Verification items for this drawing (mm, ordinates from the low corner). A direction names the side the tool comes from. Give positions to 0.01 mm unless a question says otherwise; leave off trailing zeros. Loops run counter-clockwise (first coordinate to the right, second up) from the corner with the lowest first, then second, coordinate; pieces in that order, holes last. Notation, with made-up numbers: (51.25, -15) -> (82.25, -15) arc R20 cw to (82.25, 6) -> close; hole circle Ø7 at (-32.5, 9.25). An arc over 180 degrees is marked (long way). Write item = value, one per line.
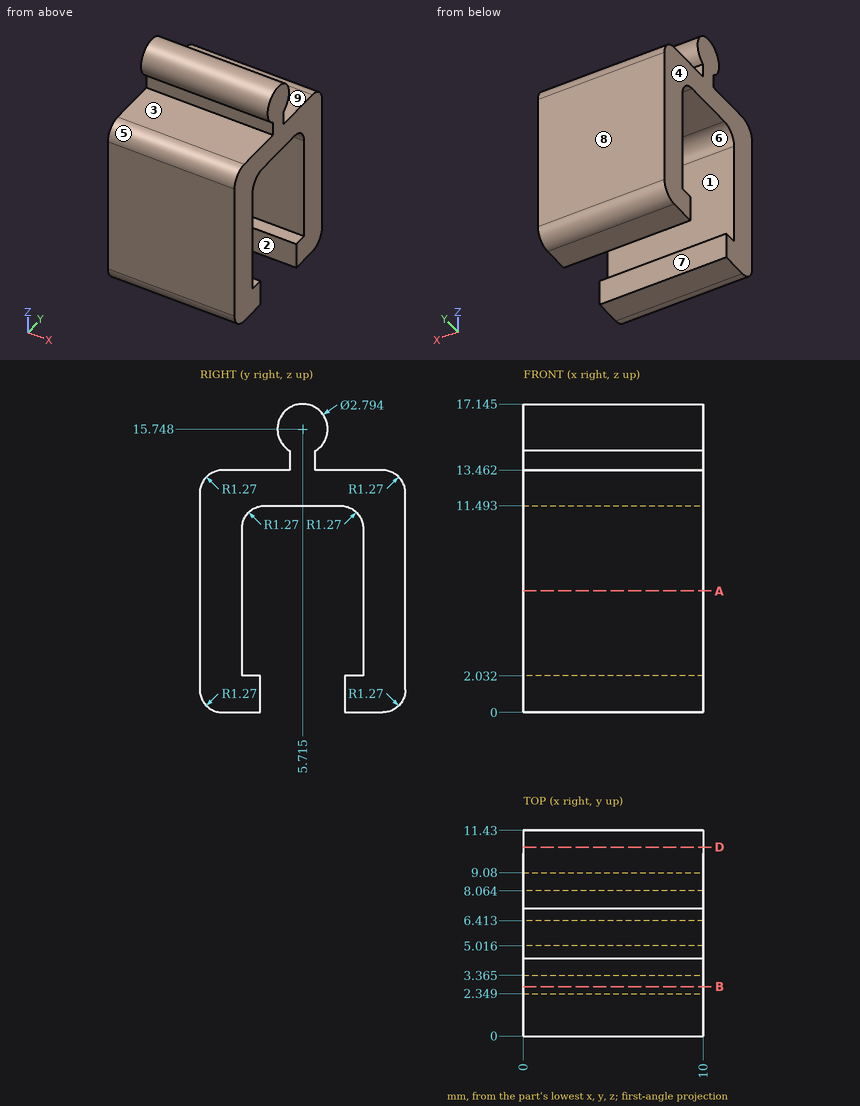
Item 1: Draft check along Y on the marked faces 6, 7, 8 and 9. Enter one of: +Y half, -Y half, draft (parallel to the pull), parting line (faces both ways), or undercut.
Answer:
face_6 = undercut
face_7 = undercut
face_8 = +Y half
face_9 = draft
Item 2: Gauge pin test, flat ends, axial feed: pin 1 (2 mm diameter, centred on x = 9, y = 7.5, fed in from +Z) (1 decimal); pin 2 (1.3 mm diameter, centred on x = 6, y = 6, fed in from -Z); pin 3 (1.1 mm diameter, centred on x = 7.5, y = 2.5, fed in from +Z); pin 4 (6 mm diameter, centred on y = 4.5, z = 11.5, fed in from -X). Record the tip position at first contact, or that the pin passes through.
Answer:
pin_1 = 16.9
pin_2 = 11.49
pin_3 = 13.46
pin_4 = 0
Item 3: Thickness scan on L1, parallel to Y at x = 5, z = 5.75; L2, parallel to Y at x = 5.25, z = 1.5 (1 decimal); L3, parallel to Z at x = 4.75, y = 9.5. Record the ranges inside material, lowest first. Write a range as [from, to].
Answer:
L1 = [0, 2.35], [9.08, 11.43]
L2 = [0, 3.4], [8.1, 11.4]
L3 = [0, 13.46]
Item 4: Section check D-D, the plane y = 10.5. Record the cut outline in (x, z) (1 decimal), plus the area to 3 significant figures.
Answer:
outline = (0, 0) -> (10, 0) -> (10, 13.4) -> (0, 13.4) -> close
area = 134 mm^2
Item 5: Tool access check on the marked faces 1, 2, 3, 4 and 5. Record the directions out of +Z, -Z, +X, -X, +Y, -Y that give a thin tool (end or side, any length) a straight path to the whole face; none if there is none.
Answer:
face_1 = +X, -X
face_2 = -Z, +X, -X
face_3 = +X, -X, -Y
face_4 = +Z, -Z, -X, +Y, -Y
face_5 = +Z, +X, -X, -Y
Item 6: Section check A-A, the plane z = 6.75. Record the cut outline in (x, y).
Answer:
outline = (0, 0) -> (10, 0) -> (10, 2.35) -> (0, 2.35) -> close; (0, 9.08) -> (10, 9.08) -> (10, 11.43) -> (0, 11.43) -> close
Item 7: Section check B-B, the plane y = 2.75. Record the cut outline in (x, z).
Answer:
outline = (0, 0) -> (10, 0) -> (10, 2.03) -> (0, 2.03) -> close; (0, 11.15) -> (10, 11.15) -> (10, 13.46) -> (0, 13.46) -> close
